from build123d import *

# Parameters (mm, degrees)
F0_W      = 15
F0_H      = 15
F1_DEPTH  = 15
F2_R      = 2
F3_R      = 1.25
F4_DEPTH  = 0.5
F7_R      = 1.25
F8_DEPTH  = 0.5
F9_DEPTH  = 1
F6_R      = 1.25
F10_DEPTH = 0.5
F11_R     = 1.25
F12_DEPTH = 0.5
F5_R      = 1.25
F13_DEPTH = 0.5
F14_R     = 1.25
F15_DEPTH = 0.5


with BuildPart() as f1:
    # F0 (on Top) → F1 (new body)
    with BuildSketch(Plane.XY):
        with Locations((-7.5, 7.5)):
            Rectangle(F0_W, F0_H)
    extrude(amount=F1_DEPTH)

    # F2
    f2_edges = [f1.edges().sort_by_distance(p)[0] for p in [
        (-15, 15, 7.5),
        (0, 15, 7.5),
        (0, 0, 7.5),
        (-7.5, 0, 15),
        (-7.5, 15, 0),
        (-7.5, 15, 15),
        (-15, 0, 7.5),
        (-7.5, 0, 0),
        (0, 7.5, 0),
        (0, 7.5, 15),
        (-15, 7.5, 0),
        (-15, 7.5, 15),
    ]]
    fillet(f2_edges, radius=F2_R)

    # F3 (on face) → F4 (cut)
    with BuildSketch(Plane.XY.offset(15)):
        with Locations((-7.5, 7.5)):
            Circle(F3_R)
    extrude(amount=-F4_DEPTH, mode=Mode.SUBTRACT)

    # F7 (on face) → F8 (join)
    with BuildSketch(Plane(origin=(-15, 0, 0), x_dir=(0, -1, 0), z_dir=(-1, 0, 0))):
        with Locations((-10.6819805153, 4.3180194847)):
            Circle(F7_R)
        with Locations((-7.5, 7.5)):
            Circle(F7_R)
        with Locations((-4.3180194847, 10.6819805153)):
            Circle(F7_R)
    extrude(amount=F8_DEPTH)

    # F9 (cut): faces of the model
    f9_faces = [f1.faces().sort_by_distance(p)[0] for p in [
        (-15.5, 10.6819805153, 4.3180194847),
        (-15.5, 7.5, 7.5),
        (-15.5, 4.3180194847, 10.6819805153),
    ]]
    extrude(f9_faces, amount=-F9_DEPTH, mode=Mode.SUBTRACT)

    # F6 (on face) → F10 (cut)
    with BuildSketch(Plane.XZ):
        with Locations((-4.5, 4.5)):
            Circle(F6_R)
        with Locations((-10.5, 4.5)):
            Circle(F6_R)
        with Locations((-10.5, 10.5)):
            Circle(F6_R)
        with Locations((-4.5, 10.5)):
            Circle(F6_R)
    extrude(amount=-F10_DEPTH, mode=Mode.SUBTRACT)

    # F11 (on face) → F12 (cut)
    with BuildSketch(Plane.YZ):
        with Locations((4.3180194847, 10.6819805153)):
            Circle(F11_R)
        with Locations((10.6819805153, 10.6819805153)):
            Circle(F11_R)
        with Locations((7.5, 7.5)):
            Circle(F11_R)
        with Locations((4.3180194847, 4.3180194847)):
            Circle(F11_R)
        with Locations((10.6819805153, 4.3180194847)):
            Circle(F11_R)
    extrude(amount=-F12_DEPTH, mode=Mode.SUBTRACT)

    # F5 (on face) → F13 (cut)
    with BuildSketch(Plane(origin=(0, 0, 0), x_dir=(1, 0, 0), z_dir=(0, 0, -1))):
        with Locations((-11, -4.5)):
            Circle(F5_R)
        with Locations((-7.5, -4.5)):
            Circle(F5_R)
        with Locations((-4, -4.5)):
            Circle(F5_R)
        with Locations((-4, -10.5)):
            Circle(F5_R)
        with Locations((-7.5, -10.5)):
            Circle(F5_R)
        with Locations((-11, -10.5)):
            Circle(F5_R)
    extrude(amount=-F13_DEPTH, mode=Mode.SUBTRACT)

    # F14 (on face) → F15 (cut)
    with BuildSketch(Plane(origin=(0, 15, 0), x_dir=(-1, 0, 0), z_dir=(0, 1, 0))):
        with Locations((10.5, 10.5)):
            Circle(F14_R)
        with Locations((4.5, 4.5)):
            Circle(F14_R)
    extrude(amount=-F15_DEPTH, mode=Mode.SUBTRACT)


solid = f1.part
Source: CAD feature listing. Evaluate the final solid. Frame: model axes, mm. A direction names the side the tool comes from. Give positions to 0.01 mm unless a question says otherwise; leave off trailing zeros. Loops run counter-clockwise (first coordinate to the right, second up) from the corner with the lowest first, then second, coordinate; pieces in that order, holes last. Notation, with made-up numbers: (62.5, 2) -> (97.5, 2) arc R25 ccw to (97.5, 30) -> close; hole circle Ø5 at (13.5, 28.5). An arc over 180 degrees is marked (long way). Use a Markdown table: item, result. Add a question column.
1) Pull-direction query (Y, two-part tool) for faces 6 (the face through (-7.42, 0.57, 0.6)), 7 (the face through (-11, 4, 0.5)), 8 (the face through (-8, 8, 0)); classes: +Y half, -Y half, draft (parallel to the pull), parting line (faces both ways), or undercut.
2) Reachability of faces 1 (the face through (-14.5, 4, 11)), 2 (the face through (-9.579, 14.754, 11.345)), 3 (the face through (-4, 10, 0.5)), 4 (the face through (-11, 0.5, 11)), 5 (the face through (-0.246, 11.874, 11.057)) from +Z, -Z, +X, -X, +Y, -Y: full face, straight path, thin tool, end or side. Return the list, or none.
3) First-contact query: pin 1 (1.5 mm diameter, centred on x = -10.5, z = 10.5, fed in from +Y); pin 2 (1.2 mm diameter, centred on x = -10.5, z = 4.5, fed in from -Y); pin 3 (2 mm diameter, centred on x = -7.5, y = 10.5, fed in from -Z). Flat tips, straight axial feed; report the tip coordinate or a pass-through.
4) Section query A-A, the plane x = -12.5. Return the cut outline in (y, z), then the cut area to 3 significant figures.
5) Section query D-D, the plane x = -1. Return the cut outline in (y, z), then the cut area to 3 significant figures.
6) Line query: line 1 along Y through (x, z) = (-4, 0.3); line 2 along Z through (x, y) = (-7.5, 6.5); line 3 along X through (y, z) = (11.25, 3.75). Output: solid intervals per line, ascending. Write a range as [from, to].
Numbers:
| question | item | result |
|---|---|---|
| 1 | face 6 | -Y half |
| 1 | face 7 | undercut |
| 1 | face 8 | draft |
| 2 | face 1 | -X |
| 2 | face 2 | +Y |
| 2 | face 3 | -Z |
| 2 | face 4 | -Y |
| 2 | face 5 | +X |
| 3 | pin 1 | stops at y = 14.5 |
| 3 | pin 2 | stops at y = 0.5 |
| 3 | pin 3 | stops at z = 0.5 |
| 4 | outline | (0, 2) arc R2 ccw to (2, 0) -> (13, 0) arc R2 ccw to (15, 2) -> (15, 13) arc R2 ccw to (13, 15) -> (2, 15) arc R2 ccw to (0, 13) -> close |
| 4 | area | 222 mm2 |
| 5 | outline | (0.27, 2) arc R1.73 ccw to (2, 0.27) -> (13, 0.27) arc R1.73 ccw to (14.73, 2) -> (14.73, 13) arc R1.73 ccw to (13, 14.73) -> (2, 14.73) arc R1.73 ccw to (0.27, 13) -> close |
| 5 | area | 207 mm2 |
| 6 | line 1 | y = [0.95, 3.25], [5.75, 9.25], [11.75, 14.05] |
| 6 | line 2 | z = [0, 14.5] |
| 6 | line 3 | x = [-14.5, -0.5] |
